Verification items for the finished model (mm, model axes). Face numbers are marked on the shaded views. A direction names the side the tool comes from. Give positions to 0.01 mm unless a question says otherwise; leave off trailing zeros. Order: outer loops, then holes, each group sorted by start corner. A loop starts at its lowest first (then second) coordinate and runs counter-clockwise, first axis right, second up.
Autodesk Fusion 360 part; units mm, degrees
sketch "Sketch2" plane through (0, 0, 0) normal (0, 0, 1) x (1, 0, 0)
  line L0 (-2.4, 2.5) -> (2.4, 2.5)
  line L1 (2.4, 2.5) -> (2.4, -2.5)
  line L2 (2.4, -2.5) -> (-2.4, -2.5)
  line L3 (-2.4, -2.5) -> (-2.4, 2.5)
  line L4 (-0.4, -0.8) -> (0.4, -0.8)
  line L5 (0.4, -0.8) -> (0.4, 0.8)
  line L6 (0.4, 0.8) -> (-0.4, 0.8)
  line L7 (-0.4, 0.8) -> (-0.4, -0.8)
  line L8 (0, 2.5) -> (0, -2.5) construction
  line L9 (-0.4, 0) -> (0.4, 0) construction
  line L10 (2.4, 2.5) -> (3.9, 2.5)
  line L11 (3.9, 2.5) -> (3.9, 1)
  line L12 (3.9, 1) -> (2.4, 1)
  line L13 (2.4, 1) -> (2.4, 2.5)
  line L14 (2.4, -2.5) -> (3.9, -2.5)
  line L15 (3.9, -2.5) -> (3.9, -1)
  line L16 (3.9, -1) -> (2.4, -1)
  line L17 (2.4, -1) -> (2.4, -2.5)
  line L18 (2.4, 1) -> (-2.4, 1)
  line L19 (2.4, -1) -> (-2.4, -1)
  dimension "d26" = 1.6
  dimension "d28" = 0.8
  dimension "d38" = 5
  dimension "d41" = 2
  dimension "d42" = 1.5
  dimension "d43" = 1.5
extrude "Extrude5" add sketch "Sketch2" along normal blind 2
chamfer "Chamfer1" distance 0.5 angle 45 12 edges at (0.4, 0, 0) (-0.4, 0, 0) (0, 0.8, 0) (0, 0.8, 2) (0, -0.8, 0) (0, -0.8, 2) (0.4, 0, 2) (-0.4, 0, 2) (2.4, 0, 0) (2.4, 0, 2) (-2.4, 0, 2) (-2.4, 0, 0)
equation "wire_spacing = 0.8 mm"
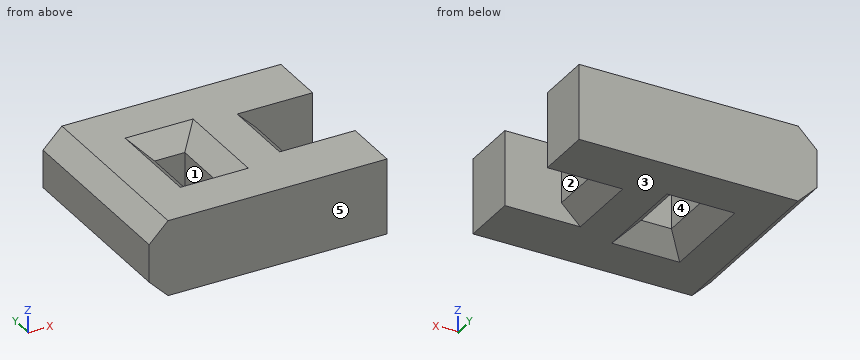
(1) Scan lines: line 1 (Y direction, x = 3.75, z = 0.25); line 2 (X direction, y = 0.5, z = 1.2); line 3 (Y direction, x = 0.25, z = 1.2). Record each from-to range of solid material in increasing order.
Solved:
line 1: y = -2.5 to -1, 1 to 2.5
line 2: x = -2.4 to -0.4, 0.4 to 2.4
line 3: y = -2.5 to -0.8, 0.8 to 2.5
(2) Section check A-A, the plane y = -0.2. Enter the section's corners in (x, z).
Solved:
outline: (-2.4, 0.5) - (-1.9, 0) - (-0.9, 0) - (-0.4, 0.5) - (-0.4, 1.5) - (-0.9, 2) - (-1.9, 2) - (-2.4, 1.5) - close; (0.4, 0.5) - (0.9, 0) - (1.9, 0) - (2.4, 0.5) - (2.4, 1.5) - (1.9, 2) - (0.9, 2) - (0.4, 1.5) - close
(3) Section check C-C, the plane z = 1.4. Enter the section's corners in (x, y), then the cut area to 3 significant figures.
Solved:
outline: (-2.4, -2.5) - (3.9, -2.5) - (3.9, -1) - (2.4, -1) - (2.4, 1) - (3.9, 1) - (3.9, 2.5) - (-2.4, 2.5) - close; hole (-0.4, -0.8) - (0.4, -0.8) - (0.4, 0.8) - (-0.4, 0.8) - close
area: 27.2 mm2
(4) Go/stop test with a flat-tipped pin: pin 1 (1.1 mm diameter, centred on y = 0, z = 1, fed in from +X). Record where the tip stops, or that it passes through.
Solved:
pin 1: stops at x = 2.4
(5) Release check for a two-part mould opening along X. For the marked faces 1, 2 and 3 record: pulls with the +X half, pulls with the -X half, needs draft (parallel to the pull), parting line crosses it, or undercut.
Solved:
face 1: undercut
face 2: pulls with the +X half
face 3: needs draft
(6) Section check B-B, the plane x = 0. Enter the section's corners in (y, z), then the cut area to 3 significant figures.
Solved:
outline: (-2.5, 0) - (-1.3, 0) - (-0.8, 0.5) - (-0.8, 1.5) - (-1.3, 2) - (-2.5, 2) - close; (0.8, 0.5) - (1.3, 0) - (2.5, 0) - (2.5, 2) - (1.3, 2) - (0.8, 1.5) - close
area: 6.30 mm2
(7) Section check D-D, the plane y = 0.9. Enter the section's corners in (x, z), then the cut area to 3 significant figures.
Solved:
outline: (-2.4, 0.5) - (-1.9, 0) - (-0.9, 0) - (-0.5, 0.4) - (0.5, 0.4) - (0.9, 0) - (1.9, 0) - (2.4, 0.5) - (2.4, 1.5) - (1.9, 2) - (0.9, 2) - (0.5, 1.6) - (-0.5, 1.6) - (-0.9, 2) - (-1.9, 2) - (-2.4, 1.5) - close
area: 7.98 mm2
(8) Set-up check for the marked faces 4 and 5: record each of +Z, -Z, +X, -X, +Y, -Y from which the full face is reachable in a straight line by a thin tool's end or side.
Solved:
face 4: +Z, -Z
face 5: +Z, -Z, +X, -X, -Y
